Geometry: final body of the model. Coordinates: model frame, mm. Round coordinates to 2 decimals unless told otherwise and drop trailing zeros. Write each loop counter-clockwise with the first axis right and the second up, starting at its lowest first coordinate (ties: lowest second). Pieces come first, ordered by that corner, then holes.
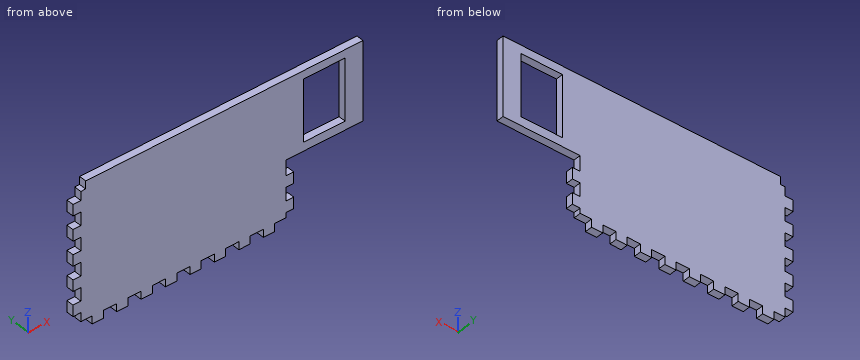
from build123d import *

# Parameters (mm, degrees)
BOSS_EXTRUDE3_DEPTH = 3
SKETCH2_W           = 17
SKETCH2_H           = 25.1
CUT_EXTRUDE1_DEPTH  = 3


with BuildPart() as part:
    # Sketch1 → Boss-Extrude3 (new body)
    with BuildSketch(Plane(origin=(0, 0, 0), x_dir=(1, 0, 0), z_dir=(0, 1, 0))):
        Polygon((-28.897216547, -2.282245917), (-28.897216547, -7.679745917), (-32.097216547, -7.679745917), (-32.097216547, -12.279745917), (-28.897216547, -12.279745917), (-28.897216547, -15.869745917), (-26.897216547, -15.869745917), (-26.897216547, -19.069745917), (55.002783453, -19.069745917), (86.572783453, -19.069745917), (86.572783453, 12.930254083), (55.002783453, 12.930254083), (55.002783453, 19.200254083), (58.202783453, 19.200254083), (58.202783453, 23.800254083), (55.002783453, 23.800254083), (55.002783453, 29.200254083), (58.202783453, 29.200254083), (58.202783453, 33.800254083), (55.002783453, 33.800254083), (55.002783453, 35.900254083), (50.352783453, 35.900254083), (50.352783453, 39.100254083), (45.752783453, 39.100254083), (45.752783453, 35.900254083), (40.352783453, 35.900254083), (40.352783453, 39.100254083), (35.752783453, 39.100254083), (35.752783453, 35.900254083), (30.352783453, 35.900254083), (30.352783453, 39.100254083), (25.752783453, 39.100254083), (25.752783453, 35.900254083), (20.352783453, 35.900254083), (20.352783453, 39.100254083), (15.752783453, 39.100254083), (15.752783453, 35.900254083), (10.352783453, 35.900254083), (10.352783453, 39.100254083), (5.752783453, 39.100254083), (5.752783453, 35.900254083), (0.352783453, 35.900254083), (0.352783453, 39.100254083), (-4.247216547, 39.100254083), (-4.247216547, 35.900254083), (-9.647216547, 35.900254083), (-9.647216547, 39.100254083), (-14.247216547, 39.100254083), (-14.247216547, 35.900254083), (-19.647216547, 35.900254083), (-19.647216547, 39.100254083), (-24.247216547, 39.100254083), (-24.247216547, 35.900254083), (-28.897216547, 35.900254083), (-28.897216547, 32.310254083), (-32.097216547, 32.310254083), (-32.097216547, 27.710254083), (-28.897216547, 27.710254083), (-28.897216547, 22.312754083), (-32.097216547, 22.312754083), (-32.097216547, 17.712754083), (-28.897216547, 17.712754083), (-28.897216547, 12.315254083), (-32.097216547, 12.315254083), (-32.097216547, 7.715254083), (-28.897216547, 7.715254083), (-28.897216547, 2.317754083), (-32.097216547, 2.317754083), (-32.097216547, -2.282245917), align=None)
    extrude(amount=BOSS_EXTRUDE3_DEPTH)

    # Sketch2 → Cut-Extrude1 (cut)
    with BuildSketch(Plane(origin=(0, 3, 0), x_dir=(1, 0, 0), z_dir=(0, 1, 0))):
        with Locations((70.732783453, -3.179745917)):
            Rectangle(SKETCH2_W, SKETCH2_H)
    extrude(amount=-CUT_EXTRUDE1_DEPTH, mode=Mode.SUBTRACT)


solid = part.part
1) Section A-A on x = 65. Output: boundary loops of the cut face in (y, z), plus the area to 3 significant figures.
2) Section C-C on x = 24.5. Output: boundary loops of the cut face in (y, z).
3) First-contact query: P1, Ø0.9, axis at x = -30.5, y = 1.5, coming from the -Z side; P2, Ø0.9, axis at y = 1.5, z = 13.5, coming from the -X side; P3, Ø1.5, axis at x = -30.5, y = 1, coming from the +Z side. Flat tips, straight axial feed; report the tip coordinate or a pass-through.
4) Line query: probe 1 along Z at (x, y) = (67.5, 2.25); probe 2 along X at (y, z) = (0.2, -5); probe 3 along X at (y, z) = (0.6, 8). Output: solid intervals per line, ascending.
5) Section B-B on z = -6.5. Output: boundary loops of the cut face in (x, y), plus the area to 3 significant figures.
Filled in:
1. outline: (0, -12.93) - (3, -12.93) - (3, -9.37) - (0, -9.37) - close; (0, 15.73) - (3, 15.73) - (3, 19.07) - (0, 19.07) - close
1. area: 20.7 mm2
2. outline: (0, -35.9) - (3, -35.9) - (3, 19.07) - (0, 19.07) - close
3. P1: stops at z = -32.31
3. P2: stops at x = -28.9
3. P3: stops at z = 12.28
4. probe 1: z = -12.93 to -9.37, 15.73 to 19.07
4. probe 2: x = -28.9 to 62.23, 79.23 to 86.57
4. probe 3: x = -32.1 to 62.23, 79.23 to 86.57
5. outline: (-28.9, 0) - (62.23, 0) - (62.23, 3) - (-28.9, 3) - close; (79.23, 0) - (86.57, 0) - (86.57, 3) - (79.23, 3) - close
5. area: 295 mm2
